The model under review builds one solid part; all positions refer to its coordinate system, in mm. Coordinates: 2 decimals unless noted, no trailing zeros. Loops run counter-clockwise (first coordinate to the right, second up) from the corner with the lowest first, then second, coordinate; pieces in that order, holes last. Notation, with made-up numbers: (40, 26) - (56, 26) arc R16 ccw to (56, 54) - close; hole circle Ø1 at (58.5, 43.25). An arc over 180 degrees is marked (long way). Answer in a Markdown table with one row per item. Add a question column.
(1) We need section D-D on x = 24. Write out the cut boundary in (y, z), plus the area to 3 significant figures.
(2) We need section A-A on x = 0. Write out the cut boundary in (y, z), plus the area to 3 significant figures.
(3) For line 1 along X through (y, z) = (1.2, 0); line 2 along Z through (x, y) = (-0.5, 1.65); line 3 along Z through (x, y) = (23.5, 0.1), list the stretches that pass through material, from the lowest coordinate up.
(4) We need section C-C on z = 5. Write out the cut boundary in (x, y), plus the area to 3 significant figures.
(5) We need section B-B on y = 2.55. Write out the cut boundary in (x, z), plus the area to 3 significant figures.
(6) For P1, Ø1, axis at y = 1.5, z = -11, coming from the -X side; P2, Ø1, axis at x = -15, z = 4.5, coming from the +Y side; P3, Ø1.5, axis at x = 9, y = 1.5, coming from the +Z side, all flat-tipped, find the tip position at first contact; note any pin that passes through.
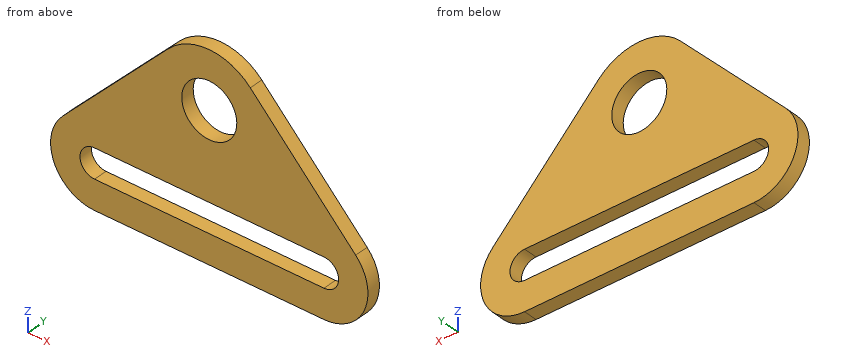
from build123d import *

# Parameters (mm, degrees)
SKETCH1_R           = 6
BOSS_EXTRUDE1_DEPTH = 3


with BuildPart() as part:
    # Sketch1 → Boss-Extrude1 (new body)
    with BuildSketch(Plane(origin=(0, 0, 0), x_dir=(1, 0, 0), z_dir=(0, 1, 0))):
        with BuildLine():
            Line((25, 31.568910727), (-25, 31.568910727))
            ThreePointArc((-25, 31.568910727), (-33.816672086, 25.743188919), (-31.915264344, 15.348123269))
            Line((-31.915264344, 15.348123269), (-8.946703241, -8.585831417))
            ThreePointArc((-8.946703241, -8.585831417), (0, -12.4), (8.946703241, -8.585831417))
            Line((8.946703241, -8.585831417), (31.915264344, 15.348123269))
            ThreePointArc((31.915264344, 15.348123269), (33.816672086, 25.743188919), (25, 31.568910727))
        make_face()
        with Locations(Location((0, 0, 0), (0, 0, 270))):
            Circle(SKETCH1_R, mode=Mode.SUBTRACT)
        with BuildLine():
            Line((-25, 25.168910727), (25, 25.168910727))
            ThreePointArc((25, 25.168910727), (28.184455364, 21.984455364), (25, 18.8))
            Line((25, 18.8), (-25, 18.8))
            ThreePointArc((-25, 18.8), (-28.184455364, 21.984455364), (-25, 25.168910727))
        make_face(mode=Mode.SUBTRACT)
    extrude(amount=BOSS_EXTRUDE1_DEPTH)


solid = part.part
Outcome:
| question | item | result |
|---|---|---|
| 1 | outline | (0, -31.57) - (3, -31.57) - (3, -25.17) - (0, -25.17) - close; (0, -18.8) - (3, -18.8) - (3, -7.1) - (0, -7.1) - close |
| 1 | area | 54.3 mm² |
| 2 | outline | (0, -31.57) - (3, -31.57) - (3, -25.17) - (0, -25.17) - close; (0, -18.8) - (3, -18.8) - (3, -6) - (0, -6) - close; (0, 6) - (3, 6) - (3, 12.4) - (0, 12.4) - close |
| 2 | area | 76.8 mm² |
| 3 | line 1 | -17.19 to -6, 6 to 17.19 |
| 3 | line 2 | -31.57 to -25.17, -18.8 to -5.98, 5.98 to 12.39 |
| 3 | line 3 | -31.57 to -25.17, -18.8 to -6.58 |
| 4 | outline | (-12.39, 0) - (-3.32, 0) - (-3.32, 3) - (-12.39, 3) - close; (3.32, 0) - (12.39, 0) - (12.39, 3) - (3.32, 3) - close |
| 4 | area | 54.4 mm² |
| 5 | outline | (-31.92, -15.35) arc R9.58 ccw to (-25, -31.57) - (25, -31.57) arc R9.58 ccw to (31.92, -15.35) - (8.95, 8.59) arc R12.4 ccw to (-8.95, 8.59) - close; hole (-25, -25.17) - (25, -25.17) arc R3.18 ccw to (25, -18.8) - (-25, -18.8) arc R3.18 ccw to start; hole circle Ø12 at (0, 0) |
| 5 | area | 1,630 mm² |
| 6 | P1 | x = -28.22 |
| 6 | P2 | through |
| 6 | P3 | z = 9.26 |
